```python
from build123d import *

# Parameters (mm, degrees)
SKETCH1_W           = 70
SKETCH1_H           = 70
BOSS_EXTRUDE1_DEPTH = 8
SKETCH3_W           = 7
SKETCH3_H           = 36


with BuildPart() as part:
    # Sketch1 → Boss-Extrude1 (new body)
    with BuildSketch(Plane(origin=(0, 0, 0), x_dir=(1, 0, 0), z_dir=(0, 1, 0))):
        Rectangle(SKETCH1_W, SKETCH1_H)
    extrude(amount=BOSS_EXTRUDE1_DEPTH)

    # Sketch3 → Revolve1 (revolve)
    with BuildSketch(Plane.XY, mode=Mode.PRIVATE) as revolve1_sk:
        with Locations((-3.5, 18)):
            Rectangle(SKETCH3_W, SKETCH3_H)
    revolve(revolve1_sk.sketch.rotate(Axis((0, -7.263286828, 0), (0, 1, 0)), 270), axis=Axis((0, -7.263286828, 0), (0, 1, 0)))


solid = part.part
```
Input: part model. Units: mm. Frame: model coordinates. A direction names the side the tool comes from. Coordinates: 2 decimals unless noted, no trailing zeros. Write each loop counter-clockwise with the first axis right and the second up, starting at its lowest first coordinate (ties: lowest second). Pieces come first, ordered by that corner, then holes.
1) Pin query (flat end, axial travel): pin 1 Ø3 at (x, z) = (23, -11.5) entering from +Y. Return the tip coordinate at first contact, or that it passes through.
2) Section C-C on y = 22. Output: boundary loops of the cut face in (x, z), and give its area (3 significant figures).
3) Section B-B on z = 0. Output: boundary loops of the cut face in (x, y), and give its area (3 significant figures).
4) Set-up query: faces 1 (the flat face through (0, 4, -35)), 2 (the cylindrical face through (6.834, 22.196, 1.517)). Return all of +Z, -Z, +X, -X, +Y, -Y with unobstructed straight access to the full face (end or side cutting, diameter ignored); none if empty.
5) Section D-D on x = 11. Output: boundary loops of the cut face in (y, z).
6) Section A-A on x = 0. Output: boundary loops of the cut face in (y, z), and give its area (3 significant figures).
7) Material intervals for line 1 along X through (y, z) = (23, 0); line 2 along Y through (x, z) = (-13, -1); line 3 along X through (y, z) = (32, 4.5), sorted ascending.
Check result:
1. pin 1: stops at y = 8
2. outline: circle Ø14 at (0, 0)
2. area: 154 mm2
3. outline: (-35, 0) - (35, 0) - (35, 8) - (7, 8) - (7, 36) - (-7, 36) - (-7, 8) - (-35, 8) - close
3. area: 952 mm2
4. face 1: -Z, +X, -X, +Y, -Y
4. face 2: +Y
5. outline: (0, -35) - (8, -35) - (8, 35) - (0, 35) - close
6. outline: (0, -35) - (8, -35) - (8, -7) - (36, -7) - (36, 7) - (8, 7) - (8, 35) - (0, 35) - close
6. area: 952 mm2
7. line 1: x = -7 to 7
7. line 2: y = 0 to 8
7. line 3: x = -5.36 to 5.36
